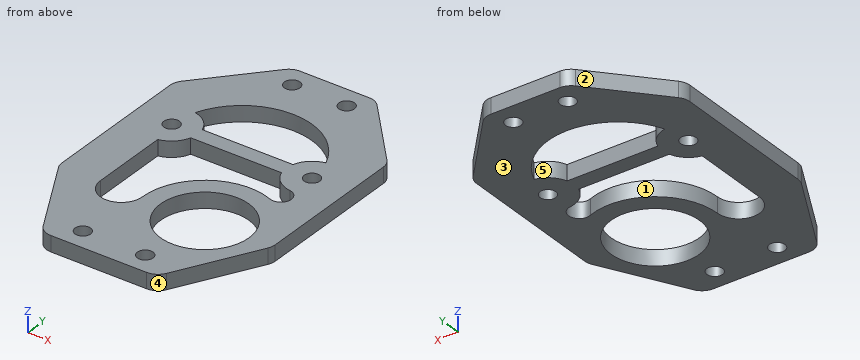
```python
from build123d import *

# Parameters (mm, degrees)
SKETCH2_R           = 1.5
SKETCH2_R_2         = 8.5
BOSS_EXTRUDE2_DEPTH = 3
FILLET1_R           = 3


with BuildPart() as part:
    # Sketch2 → Boss-Extrude2 (new body)
    with BuildSketch(Plane.XY):
        Polygon((17.549495066, -24.63349929), (-4.450504934, -24.63349929), (-13.950504934, -7.033783383), (-13.950504934, 23.266216617), (-1.440329536, 37.36650071), (14.539319668, 37.36650071), (27.049495066, 23.266216617), (27.049495066, -7.033783383), align=None)
        with Locations((1.309670464, 33.36650071)):
            Circle(SKETCH2_R, mode=Mode.SUBTRACT)
        with Locations((-6.950504934, 12.966216617)):
            Circle(SKETCH2_R, mode=Mode.SUBTRACT)
        with Locations((0.549495066, -20.63349929)):
            Circle(SKETCH2_R, mode=Mode.SUBTRACT)
        with Locations(Location((12.549495066, -20.63349929, 0), (0, 0, 180))):
            Circle(SKETCH2_R, mode=Mode.SUBTRACT)
        with Locations(Location((20.049495066, 12.966216617, 0), (0, 0, 180))):
            Circle(SKETCH2_R, mode=Mode.SUBTRACT)
        with Locations(Location((11.789319668, 33.36650071, 0), (0, 0, 180))):
            Circle(SKETCH2_R, mode=Mode.SUBTRACT)
        with Locations((14.049495066, -7.033783383)):
            Circle(SKETCH2_R_2, mode=Mode.SUBTRACT)
        with BuildLine():
            Line((-6.024579008, 8.052698409), (-6.024579008, -7.033783383))
            ThreePointArc((-6.024579008, -7.033783383), (-1.987541971, -11.07082042), (2.049495066, -7.033783383))
            ThreePointArc((2.049495066, -7.033783383), (7.232677945, 2.841995287), (18.304662454, 4.186446138))
            ThreePointArc((18.304662454, 4.186446138), (21.07880608, 5.456718839), (19.40520679, 8.007901115))
            ThreePointArc((19.40520679, 8.007901115), (16.837362911, 9.134479803), (15.279799059, 11.466216617))
            Line((15.279799059, 11.466216617), (-2.180808927, 11.466216617))
            ThreePointArc((-2.180808927, 11.466216617), (-3.63040645, 9.227641212), (-6.024579008, 8.052698409))
        make_face(mode=Mode.SUBTRACT)
        with BuildLine():
            Line((-2.180808927, 14.466216617), (15.279799059, 14.466216617))
            ThreePointArc((15.279799059, 14.466216617), (16.729396583, 16.704792022), (19.12356914, 17.879734825))
            ThreePointArc((19.12356914, 17.879734825), (6.549495066, 26.466216617), (-6.024579008, 17.879734825))
            ThreePointArc((-6.024579008, 17.879734825), (-3.63040645, 16.704792022), (-2.180808927, 14.466216617))
        make_face(mode=Mode.SUBTRACT)
    extrude(amount=BOSS_EXTRUDE2_DEPTH)

    # Fillet1
    fillet1_edges = [part.edges().sort_by_distance(p)[0] for p in [
        (-13.950504934, -7.033783383, 1.5),
        (-13.950504934, 23.266216617, 1.5),
        (-1.440329536, 37.36650071, 1.5),
        (14.539319668, 37.36650071, 1.5),
        (27.049495066, 23.266216617, 1.5),
        (27.049495066, -7.033783383, 1.5),
        (17.549495066, -24.63349929, 1.5),
        (-4.450504934, -24.63349929, 1.5),
    ]]
    fillet(fillet1_edges, radius=FILLET1_R)


solid = part.part
```
Geometry check sheet. Reference: the model listing, model coordinates, mm. Face numbers are marked on the shaded views. A direction names the side the tool comes from. Coordinates: 2 decimals unless noted, no trailing zeros. Write each loop counter-clockwise with the first axis right and the second up, starting at its lowest first coordinate (ties: lowest second). Pieces come first, ordered by that corner, then holes. Notation, with made-up numbers: M 54,62.5 L 60,62.5 A17 ccw 60,93.5 Z; hole C 14.25,58 d8. An arc over 180 degrees is marked long. Use one line per item in the form item = value. Start each with the question number.
1) Section check C-C on y = 20.5. Enter the section's corners in (x, z), and give its area (3 significant figures).
2) Thickness scan on probe 1 along Y at (x, z) = (8.5, 1.6); probe 2 along Y at (x, z) = (6.5, 2.35); probe 3 along X at (y, z) = (33.5, 0.2). Record the ranges inside material, lowest first. Write a range as from..to.
3) Section check B-B on x = 16.5. Enter the section's corners in (y, z), and give its area (3 significant figures).
4) Section check D-D on z = 0.85. State how many separate pieces and enclosed holes the cut face has, and give its area (3 significant figures).
5) Section check A-A on y = -8.5. Enter the section's corners in (x, z), and give its area (3 significant figures).
6) Set-up check for the marked faces 1 and 2: record each of +Z, -Z, +X, -X, +Y, -Y from which the full face is reachable in a straight line by a thin tool's end or side.
7) Release check for a two-part mould opening along X. For the marked faces 3, 4 and 5 record: pulls with the +X half, pulls with the -X half, needs draft (parallel to the pull), parting line crosses it, or undercut.
8) Go/stop test with a flat-tipped pin: pin 1 Ø2.5 at (x, y) = (11.79, 33.37) entering from -Z. Record where the tip stops, or that it passes through.
Responses:
q1.outline = M -13.95,0 L -4.65,0 L -4.65,3 L -13.95,3 Z; M 17.75,0 L 27.05,0 L 27.05,3 L 17.75,3 Z
q1.area = 55.8 mm2
q2.probe_1 = -24.63..-13.47, -0.6..3.61, 11.47..14.47, 26.32..37.37
q2.probe_2 = -24.63..-10.94, -3.13..2.29, 11.47..14.47, 26.47..37.37
q2.probe_3 = -4.87..-0.18, 2.8..10.3, 13.28..17.97
q3.outline = M -24.54,0 L -15.17,0 L -15.17,3 L -24.54,3 Z; M 1.11,0 L 4.71,0 L 4.71,3 L 1.11,3 Z; M 9.44,0 L 16.49,0 L 16.49,3 L 9.44,3 Z; M 22.09,0 L 35.16,0 L 35.16,3 L 22.09,3 Z
q3.area = 99.3 mm2
q4.separate_pieces = 1
q4.enclosed_holes = 9
q4.area = 1,400 mm2
q5.outline = M -13.16,0 L -5.75,0 L -5.75,3 L -13.16,3 Z; M 1.77,0 L 5.68,0 L 5.68,3 L 1.77,3 Z; M 22.42,0 L 26.26,0 L 26.26,3 L 22.42,3 Z
q5.area = 45.4 mm2
q6.face_1 = +Z, -Z
q6.face_2 = +Z, -Z, -X, +Y
q7.face_3 = needs draft
q7.face_4 = pulls with the +X half
q7.face_5 = undercut
q8.pin_1 = through
